Build history of the part. All positions in model axes, mm. Coordinates: 2 decimals unless noted, no trailing zeros. Loops run counter-clockwise (first coordinate to the right, second up) from the corner with the lowest first, then second, coordinate; pieces in that order, holes last.
Item 1: Drill centre lines: line 1 along Z through (x, y) = (0, -0.4); line 2 along X through (y, z) = (-0.55, 20); line 3 along X through (y, z) = (-0.05, 15). Where is each one in solid material? Low to high.
Item 2: Mould opens along X. For faces 1 (the face through (-3.1, -0.8, 45.1)), 2 (the face through (20.883, -0.394, 39.861)), 3 (the face through (77.77, -0.39, 207.72)), 4 (the face through (98.04, -0.394, -86.803)) say: released by +X, released by -X, zero draft, split by the parting line, or undercut.
Item 3: Cut at A-A (y = -0.3). List the corners of the cut face in (x, z), and give its area (3 significant figures).
Item 4: Cut at B-B (z = 35). List the corners of the cut face in (x, y), and give its area (3 significant figures).
Item 5: Flat gauge pin, fed straight in: pin 1 (2.5 mm diameter, centred on x = 154.23, z = -114.08, fed in from -Y). Where does the tip first touch, or does it go through?
Item 6: Cut at C-C (x = 0). List the corners of the cut face in (y, z).
Item 7: Cut at D-D (z = -21). List the corners of the cut face in (x, y), and give its area (3 significant figures).
from build123d import *

# Parameters (mm, degrees)
F3_DEPTH = 0.8
F4_R     = 1.5
F5_DEPTH = 25


with BuildPart() as f3:
    # F2 (on Front) → F3 (new body)
    with BuildSketch(Plane.XZ):
        with BuildLine():
            ThreePointArc((-45, 0), (22.035907, 39.235428), (23.418613, -38.426145))
            Line((23.418613, -38.426145), (174.780785, -136.553715))
            ThreePointArc((174.780785, -136.553715), (72.211017, 209.71602), (-221.8, 0))
            Line((-221.8, 0), (-45, 0))
        make_face()
    extrude(amount=F3_DEPTH)

    # F4 (on face) → F5 (cut)
    with BuildSketch(Plane.XZ.offset(0.8)):
        with Locations((-191.8, 10)):
            Circle(F4_R)
        with Locations((-131.8, 10)):
            Circle(F4_R)
        with Locations((-71.8, 10)):
            Circle(F4_R)
        with Locations((154.231854, -114.075886)):
            Circle(F4_R)
        with Locations((104.198704, -80.959667)):
            Circle(F4_R)
        with Locations((54.165555, -47.843448)):
            Circle(F4_R)
    extrude(amount=-F5_DEPTH, mode=Mode.SUBTRACT)


solid = f3.part
Filled sheet:
1. line 1: z = 45 to 221.8
1. line 2: x = -220.9 to -40.31, 40.31 to 220.9
1. line 3: x = -221.29 to -42.43, 42.43 to 221.29
2. face 1: zero draft
2. face 2: undercut
2. face 3: split by the parting line
2. face 4: released by -X
3. outline: (-221.8, 0) - (-45, 0) arc R45 cw (long way) to (23.42, -38.43) - (174.78, -136.55) arc R221.8 ccw (long way) to start; hole circle Ø3 at (-191.8, 10); hole circle Ø3 at (-131.8, 10); hole circle Ø3 at (-71.8, 10); hole circle Ø3 at (54.17, -47.84); hole circle Ø3 at (104.2, -80.96); hole circle Ø3 at (154.23, -114.08)
3. area: 91,100 mm2
4. outline: (-219.02, -0.8) - (-28.28, -0.8) - (-28.28, 0) - (-219.02, 0) - close; (28.28, -0.8) - (219.02, -0.8) - (219.02, 0) - (28.28, 0) - close
4. area: 305 mm2
5. pin 1: passes through
6. outline: (-0.8, 45) - (0, 45) - (0, 221.8) - (-0.8, 221.8) - close
7. outline: (39.8, -0.8) - (220.8, -0.8) - (220.8, 0) - (39.8, 0) - close
7. area: 145 mm2
